Design review of the part built by this model. Coordinates are the model's own, in mm. Face numbers are marked on the shaded views. A direction names the side the tool comes from. Coordinates: 2 decimals unless noted, no trailing zeros. Loops run counter-clockwise (first coordinate to the right, second up) from the corner with the lowest first, then second, coordinate; pieces in that order, holes last.
Q1. For P1, Ø21.5, axis at y = -42.71, z = -42.71, coming from the -X side; P2, Ø11.5, axis at y = -42.66, z = 42.66, coming from the -X side; P3, Ø15, axis at y = 42.66, z = -42.66, coming from the -X side (3 decimals); P4, Ø2, axis at x = 26.5, y = -11.5, coming from the +Z side, all flat-tipped, find the tip position at first contact; note any pin that passes through.
Q2. Draft analysis for pull direction Z (two halves, no side actions). For the marked faces 4, 5, 6 and 7, state which applies: released by +Z, released by -Z, zero draft, split by the parting line, or undercut.
Q3. Add section B-B on x = 12.5. Give the boundary of the cut face in (y, z) (3 decimals).
Q4. Add section A-A on x = 44.5. Give the boundary of the cut face in (y, z).
Q5. Wall thickness on probe 1 along X at (y, z) = (34, 30) (3 decimals); probe 2 along X at (y, z) = (-52, 34.5) (3 decimals); probe 3 along Z at (x, y) = (41.5, 1.5): over which ranges is each line inside the solid? List them lowest first.
Q6. Machinability: for the marked faces 1, 2 and 3, which of the approach directions +Z, -Z, +X, -X, +Y, -Y give a long, thin tool a straight path to every point of the face, cutting with its end or side? Answer none if there is none.
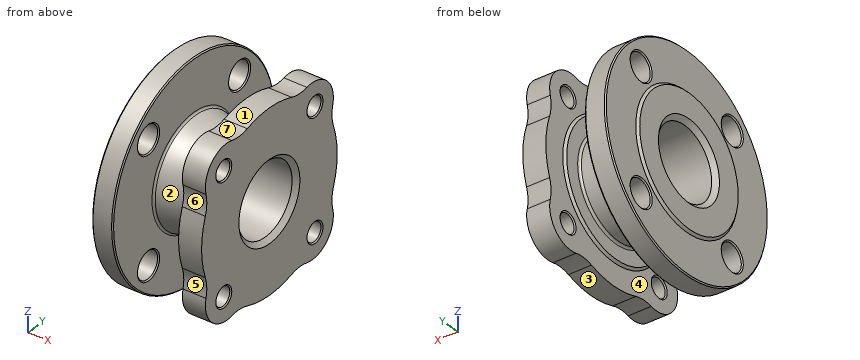
```python
from build123d import *

# Parameters (mm, degrees)
SKETCH2_R           = 6.6675
SKETCH2_R_2         = 25.4
BOSS_EXTRUDE2_DEPTH = 16.51
CUT_EXTRUDE1_REACH  = 129.898
SKETCH3_R           = 9.525
CHAMFER1_SIZE       = 0.8128
CHAMFER2_SIZE       = 3.175
FILLET1_R           = 1.524


with BuildPart() as part:
    # Sketch1 → Revolve1 (revolve)
    with BuildSketch(Plane.XY, mode=Mode.PRIVATE) as revolve1_sk:
        Polygon((0, 25.4), (53.975, 25.4), (53.975, 47.625), (52.3748, 46.0248), (52.3748, 34.29), (35.052, 34.29), (16.51, 38.231223766), (16.51, 76.2), (1.6002, 76.2), (1.6002, 47.7012), (0, 46.101), align=None)
    revolve(revolve1_sk.sketch.rotate(Axis((0, 0, 0), (1, 0, 0)), 90), axis=Axis((0, 0, 0), (1, 0, 0)))

    # Sketch2 → Boss-Extrude2 (add)
    with BuildSketch(Plane(origin=(53.975, 0, 0), x_dir=(0, 0, -1), z_dir=(1, 0, 0))):
        with BuildLine():
            ThreePointArc((-60.006129061, 20.772926495), (-63.5, 0), (-60.006129061, -20.772926495))
            ThreePointArc((-60.006129061, -20.772926495), (-58.634269802, -27.940016869), (-59.356714755, -35.20137043))
            ThreePointArc((-59.356714755, -35.20137043), (-54.10400211, -54.10400211), (-35.20137043, -59.356714755))
            ThreePointArc((-35.20137043, -59.356714755), (-27.940016869, -58.634269802), (-20.772926495, -60.006129061))
            ThreePointArc((-20.772926495, -60.006129061), (0, -63.5), (20.772926495, -60.006129061))
            ThreePointArc((20.772926495, -60.006129061), (27.940016869, -58.634269802), (35.20137043, -59.356714755))
            ThreePointArc((35.20137043, -59.356714755), (54.10400211, -54.10400211), (59.356714755, -35.20137043))
            ThreePointArc((59.356714755, -35.20137043), (58.634269802, -27.940016869), (60.006129061, -20.772926495))
            ThreePointArc((60.006129061, -20.772926495), (63.5, 0), (60.006129061, 20.772926495))
            ThreePointArc((60.006129061, 20.772926495), (58.634269802, 27.940016869), (59.356714755, 35.20137043))
            ThreePointArc((59.356714755, 35.20137043), (54.10400211, 54.10400211), (35.20137043, 59.356714755))
            ThreePointArc((35.20137043, 59.356714755), (27.940016869, 58.634269802), (20.772926495, 60.006129061))
            ThreePointArc((20.772926495, 60.006129061), (0, 63.5), (-20.772926495, 60.006129061))
            ThreePointArc((-20.772926495, 60.006129061), (-27.940016869, 58.634269802), (-35.20137043, 59.356714755))
            ThreePointArc((-35.20137043, 59.356714755), (-54.10400211, 54.10400211), (-59.356714755, 35.20137043))
            ThreePointArc((-59.356714755, 35.20137043), (-58.634269802, 27.940016869), (-60.006129061, 20.772926495))
        make_face()
        with Locations((-42.706424702, 42.706424702)):
            Circle(SKETCH2_R, mode=Mode.SUBTRACT)
        with Locations(Location((42.706424702, 42.706424702, 0), (0, 0, 180))):
            Circle(SKETCH2_R, mode=Mode.SUBTRACT)
        with Locations((42.706424702, -42.706424702)):
            Circle(SKETCH2_R, mode=Mode.SUBTRACT)
        with Locations(Location((-42.706424702, -42.706424702, 0), (0, 0, 180))):
            Circle(SKETCH2_R, mode=Mode.SUBTRACT)
        with Locations(Location((0, 0, 0), (0, 0, 180))):
            Circle(SKETCH2_R_2, mode=Mode.SUBTRACT)
    extrude(amount=BOSS_EXTRUDE2_DEPTH)

    # Sketch3 → Cut-Extrude1 (cut, up to next)
    with BuildSketch(Plane.ZY.offset(-1.6002), mode=Mode.PRIVATE) as cut_extrude1_sk1:
        with Locations((42.656216575, 42.656216575)):
            Circle(SKETCH3_R)
    cut_extrude1_tool1 = extrude(cut_extrude1_sk1.sketch, amount=-CUT_EXTRUDE1_REACH, mode=Mode.PRIVATE) & part.part
    # Sketch3 → Cut-Extrude1 (cut, up to next)
    with BuildSketch(Plane.ZY.offset(-1.6002), mode=Mode.PRIVATE) as cut_extrude1_sk2:
        with Locations((-42.656216575, 42.656216575)):
            Circle(SKETCH3_R)
    cut_extrude1_tool2 = extrude(cut_extrude1_sk2.sketch, amount=-CUT_EXTRUDE1_REACH, mode=Mode.PRIVATE) & part.part
    # Sketch3 → Cut-Extrude1 (cut, up to next)
    with BuildSketch(Plane.ZY.offset(-1.6002), mode=Mode.PRIVATE) as cut_extrude1_sk3:
        with Locations((42.656216575, -42.656216575)):
            Circle(SKETCH3_R)
    cut_extrude1_tool3 = extrude(cut_extrude1_sk3.sketch, amount=-CUT_EXTRUDE1_REACH, mode=Mode.PRIVATE) & part.part
    # Sketch3 → Cut-Extrude1 (cut, up to next)
    with BuildSketch(Plane.ZY.offset(-1.6002), mode=Mode.PRIVATE) as cut_extrude1_sk4:
        with Locations((-42.656216575, -42.656216575)):
            Circle(SKETCH3_R)
    cut_extrude1_tool4 = extrude(cut_extrude1_sk4.sketch, amount=-CUT_EXTRUDE1_REACH, mode=Mode.PRIVATE) & part.part
    add(cut_extrude1_tool1.solids().sort_by_distance((1.6002, 42.656217, 42.656217))[0], mode=Mode.SUBTRACT)
    add(cut_extrude1_tool2.solids().sort_by_distance((1.6002, 42.656217, -42.656217))[0], mode=Mode.SUBTRACT)
    add(cut_extrude1_tool3.solids().sort_by_distance((1.6002, -42.656217, 42.656217))[0], mode=Mode.SUBTRACT)
    add(cut_extrude1_tool4.solids().sort_by_distance((1.6002, -42.656217, -42.656217))[0], mode=Mode.SUBTRACT)

    # Chamfer1
    chamfer1_edges = [part.edges().sort_by_distance(p)[0] for p in [
        (53.975, -42.706424702, 36.038924702),
        (53.975, 42.706424702, -49.373924702),
        (53.975, 42.706424702, 49.373924702),
        (53.975, -42.706424702, -36.038924702),
        (70.485, 42.706424702, 49.373924702),
        (70.485, 42.706424702, -49.373924702),
        (70.485, -42.706424702, -36.038924702),
        (70.485, -42.706424702, 36.038924702),
        (1.6002, 42.656216575, 33.131216575),
        (16.51, 42.656216575, 33.131216575),
        (1.6002, 42.656216575, -52.181216575),
        (16.51, 42.656216575, -52.181216575),
        (1.6002, -42.656216575, 33.131216575),
        (16.51, -42.656216575, 33.131216575),
        (1.6002, -42.656216575, -52.181216575),
        (16.51, -42.656216575, -52.181216575),
        (1.6002, 0, -76.2),
        (16.51, 0, -76.2),
    ]]
    chamfer(chamfer1_edges, length=CHAMFER1_SIZE)

    # Chamfer2
    chamfer2_edges = [part.edges().sort_by_distance(p)[0] for p in [
        (0, 0, -25.4),
        (70.485, 0, -25.4),
    ]]
    chamfer(chamfer2_edges, length=CHAMFER2_SIZE)

    # Fillet1
    fillet1_edges = [part.edges().sort_by_distance(p)[0] for p in [
        (52.3748, 0, -34.29),
        (16.51, 0, -38.231223766),
    ]]
    fillet(fillet1_edges, radius=FILLET1_R)


solid = part.part
```
Entries:
1. P1: stops at x = 1.6
1. P2: passes through
1. P3: stops at x = 53.975
1. P4: stops at z = 34.62
2. face 4: zero draft
2. face 5: undercut
2. face 6: undercut
2. face 7: released by +Z
3. outline: circle Ø152.4 at (0, 0); hole circle Ø19.05 at (-42.656, -42.656); hole circle Ø19.05 at (-42.656, 42.656); hole circle Ø50.8 at (0, 0); hole circle Ø19.05 at (42.656, -42.656); hole circle Ø19.05 at (42.656, 42.656)
4. outline: circle Ø68.58 at (0, 0); hole circle Ø50.8 at (0, 0)
5. probe 1: x = 0 to 16.51, 52.375 to 70.485
5. probe 2: x = 1.6 to 16.51, 53.975 to 70.485
5. probe 3: z = -34.26 to -25.36, 25.36 to 34.26
6. face 1: +Z, +X
6. face 2: none
6. face 3: -Z, +X
